Source: CAD feature listing. Evaluate the final solid. Frame: model axes, mm. A direction names the side the tool comes from. Round coordinates to 2 decimals unless told otherwise and drop trailing zeros. Order: outer loops, then holes, each group sorted by start corner. A loop starts at its lowest first (then second) coordinate and runs counter-clockwise, first axis right, second up. Notation, with made-up numbers: (48.25, -35) - (80.25, -35) arc R20 cw to (80.25, 1) - close; hole circle Ø8 at (89, 29). An arc over 180 degrees is marked (long way). Return JSON: item names as keys, results as strings. Group by question number.
1) Mould query, pull axis Y, two halves, no side actions, for faces 3 (the cylindrical face through (-45.862, -26.395, -1.521)), 4 (the cylindrical face through (-42.405, -23.46, 2.465)), 5 (the flat face through (-1, 29.703, -2)). Classes: pulls with the +Y half, pulls with the -Y half, needs draft (parallel to the pull), parting line crosses it, or undercut.
2) Section B-B, the plane x = 37. Return loops of the section in (y, z), plus the area to 3 significant figures.
3) Section C-C, the plane y = 24. Return loops of the section in (x, z).
4) Section D-D, the plane x = -34. Return loops of the section in (y, z).
5) Contact query for flat-ended pins moving along their axis: P1, Ø2, axis at x = -16.5, y = -0.5, coming from the +Z side; P2, Ø1.5, axis at y = 23, z = 1.5, coming from the -X side. Output: stop coordinate, or through.
6) Section A-A, the plane z = 4. Return loops of the section in (x, y).
7) Access query for faces 1 (the cylindrical face through (42.38, -26.44, -1.52)), 2 (the cylindrical face through (-41.02, 21.657, 2.465)). Directions: +Z, -Z, +X, -X, +Y, -Y. A direction counts if a zero-diameter tool reaches every point of the face in a straight line with its end or side. Return the directions, or none.
8) Ray query, line 1 (Y direction, x = 37, z = -0.5); line 2 (Y direction, x = 37, z = 3); line 3 (Z direction, x = -29, y = -11). Return the intervals inside material, ascending. Write a range as from..to.
```python
from build123d import *

# Parameters (mm, degrees)
SKETCH_3_R       = 2.4
SKETCH_3_R_2     = 1.3
EXTRUDE_5_DEPTH  = 5.000409789
SKETCH_3_8_R     = 2.4
SKETCH_3_8_R_2   = 1.3
EXTRUDE_6_DEPTH  = 5
SKETCH_3_9_R     = 2.4
SKETCH_3_9_R_2   = 1.3
EXTRUDE_7_DEPTH  = 5
SKETCH_3_10_R    = 2.4
SKETCH_3_10_R_2  = 1.3
EXTRUDE_8_DEPTH  = 5
EXTRUDE_START    = -3
SKETCH_3_17_R    = 1.3
EXTRUDE_12_DEPTH = 3


with BuildPart() as part:
    # Sketch 3 → Extrude 5 (new body)
    with BuildSketch(Plane.XY):
        with Locations((-40.5, 24)):
            Circle(SKETCH_3_R)
        with Locations((-40.5, 24)):
            Circle(SKETCH_3_R_2, mode=Mode.SUBTRACT)
    extrude(amount=EXTRUDE_5_DEPTH)



with BuildPart() as body_2:
    # Sketch 3_8 → Extrude 6 (new body)
    with BuildSketch(Plane.XY):
        with Locations((37, 24)):
            Circle(SKETCH_3_8_R)
        with Locations((37, 24)):
            Circle(SKETCH_3_8_R_2, mode=Mode.SUBTRACT)
    extrude(amount=EXTRUDE_6_DEPTH)


with BuildPart() as body_3:
    # Sketch 3_9 → Extrude 7 (new body)
    with BuildSketch(Plane.XY):
        with Locations((37, -22)):
            Circle(SKETCH_3_9_R)
        with Locations((37, -22)):
            Circle(SKETCH_3_9_R_2, mode=Mode.SUBTRACT)
    extrude(amount=EXTRUDE_7_DEPTH)


with BuildPart() as body_4:
    # Sketch 3_10 → Extrude 8 (new body)
    with BuildSketch(Plane.XY):
        with Locations((-40.5, -22)):
            Circle(SKETCH_3_10_R)
        with Locations((-40.5, -22)):
            Circle(SKETCH_3_10_R_2, mode=Mode.SUBTRACT)
    extrude(amount=EXTRUDE_8_DEPTH)


with BuildPart() as part_1:
    add(part.part)

    add(body_2.part)  # Extrude 12 merges body 2

    add(body_3.part)  # Extrude 12 merges body 3

    add(body_4.part)  # Extrude 12 merges body 4
    # Sketch 3_17 → Extrude 12 (add)
    with BuildSketch(Plane.XY.offset(EXTRUDE_START)):
        with BuildLine():
            Line((40.282145442, 29.703068159), (-43.717854558, 29.703068159))
            ThreePointArc((-43.717854558, 29.703068159), (-45.839174902, 28.824388502), (-46.717854558, 26.703068159))
            Line((-46.717854558, 26.703068159), (-46.717854558, -24.296931841))
            ThreePointArc((-46.717854558, -24.296931841), (-45.839174902, -26.418252185), (-43.717854558, -27.296931841))
            Line((-43.717854558, -27.296931841), (40.282145442, -27.296931841))
            ThreePointArc((40.282145442, -27.296931841), (42.403465785, -26.418252185), (43.282145442, -24.296931841))
            Line((43.282145442, -24.296931841), (43.282145442, 26.703068159))
            ThreePointArc((43.282145442, 26.703068159), (42.403465785, 28.824388502), (40.282145442, 29.703068159))
        make_face()
        with Locations((37, 24)):
            Circle(SKETCH_3_17_R, mode=Mode.SUBTRACT)
        with Locations((37, -22)):
            Circle(SKETCH_3_17_R, mode=Mode.SUBTRACT)
        with Locations((-40.5, 24)):
            Circle(SKETCH_3_17_R, mode=Mode.SUBTRACT)
        with Locations((-40.5, -22)):
            Circle(SKETCH_3_17_R, mode=Mode.SUBTRACT)
    extrude(amount=EXTRUDE_12_DEPTH)


solid = part_1.part
```
Geometry check:
{
 "1": {"face 3": "pulls with the -Y half", "face 4": "undercut", "face 5": "pulls with the +Y half"},
 "2": {"outline": "(-27.3, -3) - (-23.3, -3) - (-23.3, 5) - (-24.4, 5) - (-24.4, 0) - (-27.3, 0) - close; (-20.7, -3) - (22.7, -3) - (22.7, 5) - (21.6, 5) - (21.6, 0) - (-19.6, 0) - (-19.6, 5) - (-20.7, 5) - close; (25.3, -3) - (29.7, -3) - (29.7, 0) - (26.4, 0) - (26.4, 5) - (25.3, 5) - close", "area": "177 mm2"},
 "3": {"outline": "(-46.72, -3) - (-41.8, -3) - (-41.8, 5) - (-42.9, 5) - (-42.9, 0) - (-46.72, 0) - close; (-39.2, -3) - (35.7, -3) - (35.7, 5) - (34.6, 5) - (34.6, 0) - (-38.1, 0) - (-38.1, 5) - (-39.2, 5) - close; (38.3, -3) - (43.28, -3) - (43.28, 0) - (39.4, 0) - (39.4, 5) - (38.3, 5) - close"},
 "4": {"outline": "(-27.3, -3) - (29.7, -3) - (29.7, 0) - (-27.3, 0) - close"},
 "5": {"P1": "z = 0", "P2": "x = -42.89"},
 "6": {"outline": "circle Ø4.8 at (-40.5, -22); circle Ø4.8 at (-40.5, 24); circle Ø4.8 at (37, -22); circle Ø4.8 at (37, 24); hole circle Ø2.6 at (-40.5, -22); hole circle Ø2.6 at (-40.5, 24); hole circle Ø2.6 at (37, -22); hole circle Ø2.6 at (37, 24)"},
 "7": {"face 1": "+Z, -Z, +X, -Y", "face 2": "+Z"},
 "8": {"line 1": "-27.3..-23.3, -20.7..22.7, 25.3..29.7", "line 2": "-24.4..-23.3, -20.7..-19.6, 21.6..22.7, 25.3..26.4", "line 3": "-3..0"}
}
